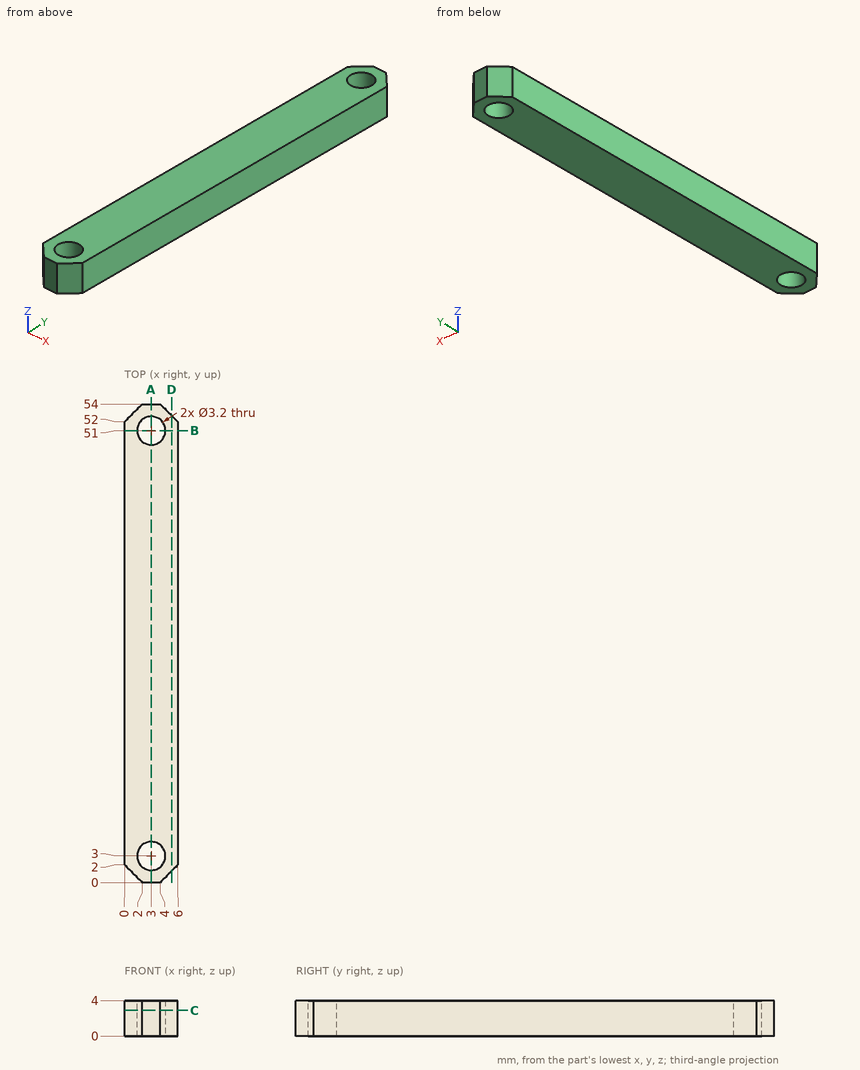
Could you check a few things on this drawing? It's one solid part, dimensions in mm from its lowest x, y, z. Round coordinates to 2 decimals unless told otherwise and drop trailing zeros. Loops run counter-clockwise (first coordinate to the right, second up) from the corner with the lowest first, then second, coordinate; pieces in that order, holes last. Notation, with made-up numbers: M 77,50 L 85,50 A29 ccw 85,75 Z; hole C -12,28.25 d2. An arc over 180 degrees is marked long. Write item = value, one per line. Start each with the question number.
(1) I'm going to push a flat-ended pin straight in: P1, Ø2, axis at x = 4.5, z = 2, coming from the +Y side. Where does the tip first touch, or does it pass through?
(2) Suppose I cut it at B-B on y = 51. Write out the boundary of the cut face in (x, z), plus the area to 3 significant figures.
(3) I need wall thicknesses on line 1 along Y through (x, z) = (3, 3.15); line 2 along Y through (x, z) = (4.15, 1.45); line 3 along Y through (x, z) = (5.55, 2.7). Which ranges of each line are inside material? Lowest first, please.
(4) Suppose I cut it at D-D on x = 5.3. Write out the boundary of the cut face in (y, z), plus the area to 3 significant figures.
(5) Suppose I cut it at A-A on x = 3. Write out the boundary of the cut face in (y, z).
(6) Suppose I cut it at C-C on z = 2.9. Write out the boundary of the cut face in (x, y), plus the area to 3 significant figures.
Answer block:
q1.P1 = 54
q2.outline = M 0,0 L 1.4,0 L 1.4,4 L 0,4 Z; M 4.6,0 L 6,0 L 6,4 L 4.6,4 Z
q2.area = 11.2 mm²
q3.line_1 = 0 to 1.4, 4.6 to 49.4, 52.6 to 54
q3.line_2 = 0.15 to 1.89, 4.11 to 49.89, 52.11 to 53.85
q3.line_3 = 1.55 to 52.45
q4.outline = M 1.3,0 L 52.7,0 L 52.7,4 L 1.3,4 Z
q4.area = 206 mm²
q5.outline = M 0,0 L 1.4,0 L 1.4,4 L 0,4 Z; M 4.6,0 L 49.4,0 L 49.4,4 L 4.6,4 Z; M 52.6,0 L 54,0 L 54,4 L 52.6,4 Z
q6.outline = M 0,2 L 2,0 L 4,0 L 6,2 L 6,52 L 4,54 L 2,54 L 0,52 Z; hole C 3,3 d3.2; hole C 3,51 d3.2
q6.area = 300 mm²
